Check sheet for the modelled part. Datum: model origin and axes. Units: mm. A direction names the side the tool comes from. Give positions to 0.01 mm unless a question says otherwise; leave off trailing zeros. Write each loop counter-clockwise with the first axis right and the second up, starting at its lowest first coordinate (ties: lowest second). Pieces come first, ordered by that corner, then holes. Notation, with made-up numbers: M -14.5,-16 L 37.5,-16 A28 ccw 37.5,10 Z; hole C 54,9 d11. An arc over 180 degrees is marked long. Use CSV: the item, a comma, the result in double quotes. Start each with the question number.
1. Depth check by flat-ended pin: P1, Ø8, axis at y = 33, z = 3, coming from the -X side; P2, Ø1, axis at x = -55, z = -1, coming from the -Y side; P3, Ø16.5, axis at y = 131, z = 0, coming from the +X side. Enter the tip coordinate at first touch or a pass-through.
2. Cross-section at B-B, the plane x = -90. Enter the section's corners in (y, z) (3 decimals), and give its area (3 significant figures).
3. Scan lines: line 1 (Z direction, x = -76.5, y = 131) (3 decimals); line 2 (Y direction, x = -68, z = 0) (3 decimals). Record each from-to range of solid material in increasing order.
4. Mould release check, pull along Z, two halves, no side actions. Record for faces 5 (the face through (-147.46, 120.51, 32.75)), 6 (the face through (-74.32, 136.89, 2.44)), 7 (the face through (-142, 126, 50)): +Z half, -Z half, draft (parallel to the pull), parting line (faces both ways), or undercut.
5. Cross-section at A-A, the plane z = 41. Enter the section's corners in (x, y) (3 decimals).
6. Access from +Z, -Z, +X, -X, +Y, -Y to the whole of each face (thin tool, end or side, straight path). Record for faces 1 (the face through (-5, 0, 5)), 2 (the face through (-74.32, 120.51, -0.46)), 3 (the face through (-144.56, 136.89, 32.75)), 4 (the face through (-1.382, 58.812, 6.223)).
from build123d import *

# Parameters (mm, degrees)
SKETCH1_R   = 10.5
SKETCH1_R_2 = 6.375


with BuildPart() as part:
    # Sweep1: sweep along a curve in space
    with BuildLine() as sweep1_path:
        Line((0, 0, 0), (0, 116, 0))
        ThreePointArc((0, 116, 0), (-4.393398282, 126.606601718, 0), (-15, 131, 0))
        Line((-15, 131, 0), (-132, 131, 0))
        ThreePointArc((-132, 131, 0), (-142.606601718, 131, 4.393398282), (-147, 131, 15))
        Line((-147, 131, 15), (-147, 131, 50))
    # Sketch1 → Sweep1 (sweep)
    with BuildSketch(Plane(origin=(0, 0, 0), x_dir=(1, 0, 0), z_dir=(0, 1, 0))):
        Circle(SKETCH1_R)
        Circle(SKETCH1_R_2, mode=Mode.SUBTRACT)
    sweep(path=sweep1_path.line)


solid = part.part
Worked answers:
1,P1,"stops at x = -10.5"
1,P2,"stops at y = 120.51"
1,P3,"stops at x = 9.59"
2,outline,"C 131,0 d21; hole C 131,0 d12.75"
2,area,"219 mm^2"
3,line 1,"z = -10.5 to -6.375, 6.375 to 10.5"
3,line 2,"y = 120.5 to 124.625, 137.375 to 141.5"
4,face 5,"draft"
4,face 6,"undercut"
4,face 7,"+Z half"
5,outline,"C -147,131 d21; hole C -147,131 d12.75"
6,face 1,"+Z, -Z, +X, -X, -Y"
6,face 2,"none"
6,face 3,"+Z"
6,face 4,"-Y"
